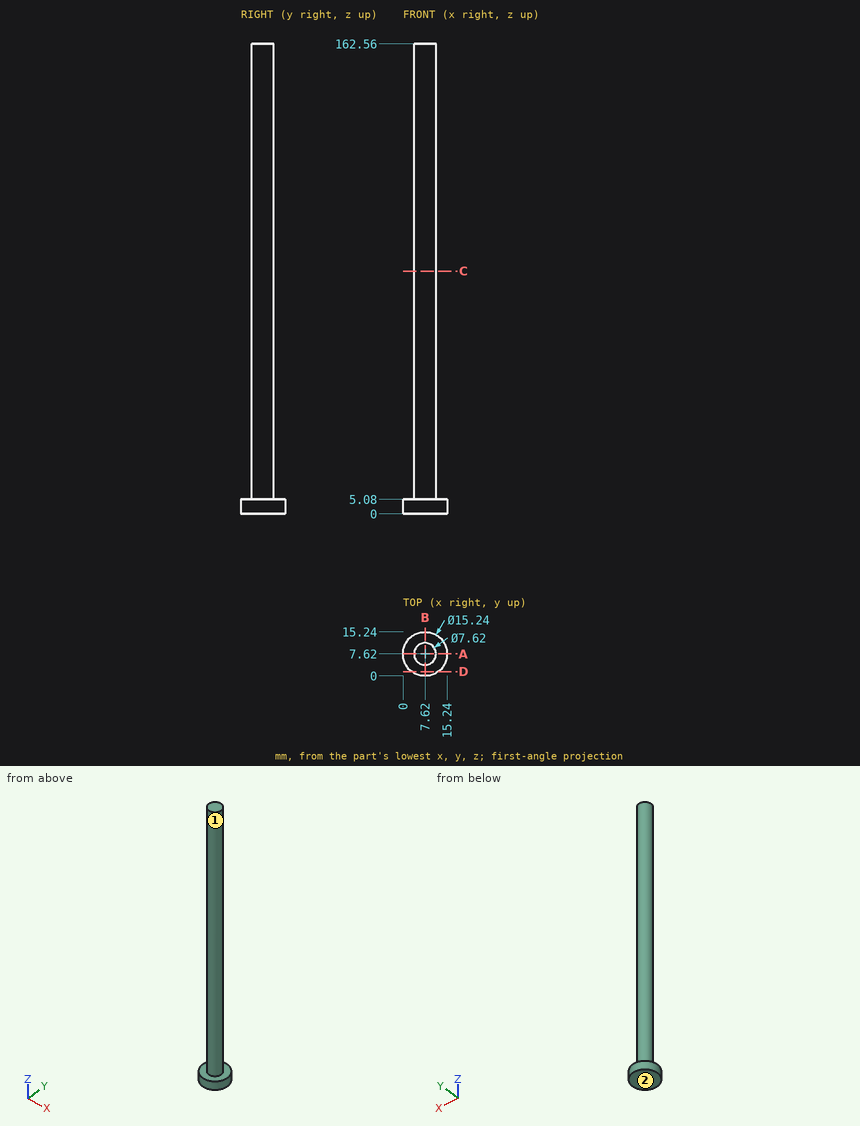
Design review of the part shown in the three views and the two pictorial views. Dimensions are in mm from the part's minimum x, y and z. A direction names the side the tool comes from. Round coordinates to 2 decimals unless told otherwise and drop trailing zeros. Loops run counter-clockwise (first coordinate to the right, second up) from the corner with the lowest first, then second, coordinate; pieces in that order, holes last. Notation, with made-up numbers: M -25.5,69.5 L -10.5,69.5 A23 cw -10.5,88.5 Z; hole C 13,81 d8. An arc over 180 degrees is marked long. Put each result on its own line as item: value.
Q1. Consider section D-D, the plane y = 1.5. Give the boundary of the cut face in (x, z), then the cut area to 3 significant figures.
Result set:
outline: M 3.08,0 L 12.16,0 L 12.16,5.08 L 3.08,5.08 Z
area: 46.1 mm²
Q2. Machinability: for the marked faces 1 and 2, which of the approach directions +Z, -Z, +X, -X, +Y, -Y give a long, thin tool a straight path to every point of the face, cutting with its end or side? Answer none if there is none.
Result set:
face 1: +Z
face 2: -Z, +X, -X, +Y, -Y
Q3. For pin 1 (5 mm diameter, centred on y = 10, z = 76, fed in from -X); pin 2 (5 mm diameter, centred on y = 12, z = 54.5, fed in from +X), all flat-tipped, find the tip position at first contact; note any pin that passes through.
Result set:
pin 1: stops at x = 3.81
pin 2: stops at x = 10.93
Q4. Consider section C-C, the plane z = 84. Give the boundary of the cut face in (x, y).
Result set:
outline: C 7.62,7.62 d7.62
Q5. To check wall thickness, follow L1, parallel to Z at x = 2.75, y = 13.25; L2, parallel to Y at x = 7.25, z = 36.5. State the ranges of each line that lie inside material, in increasing order.
Result set:
L1: z = 0 to 5.08
L2: y = 3.83 to 11.41
Q6. Consider section A-A, the plane y = 7.62. Give the boundary of the cut face in (x, z), then the cut area to 3 significant figures.
Result set:
outline: M 0,0 L 15.24,0 L 15.24,5.08 L 11.43,5.08 L 11.43,162.56 L 3.81,162.56 L 3.81,5.08 L 0,5.08 Z
area: 1,280 mm²
